Here's how the part is built. I have some questions about the finished solid (model axes, mm). A direction names the side the tool comes from. Coordinates: 2 decimals unless noted, no trailing zeros. Write each loop counter-clockwise with the first axis right and the second up, starting at its lowest first coordinate (ties: lowest second). Pieces come first, ordered by that corner, then holes.
Item 1: For faces 1 (the face through (-5, 9, 30)), 2 (the face through (-11.99, 0.53, 18.12)), 3 (the face through (0.53, 0.28, -11.99)), which set-ups out of +Z, -Z, +X, -X, +Y, -Y let a thin tool reach every point of the face, with its end or its side?
Item 2: I want a section at B-B (y = 13). Please give me the cut outline in (x, z).
Item 3: I want a section at D-D (y = 4.5). Please give me the cut outline in (x, z), and give its area (3 significant figures).
Item 4: I'm going to push flat-ended pins straight in: P1, Ø2, axis at x = 4, y = 5.5, coming from the +Z side; P2, Ø3, axis at x = -9, y = 1, coming from the -Z side; P3, Ø3, axis at x = 3.5, y = -15, coming from the -Z side; P4, Ø2, axis at x = 8.5, z = 4.5, coming from the -Y side. Where does each tip first touch, or does it pass through?
Item 5: I want a section at C-C (z = -8). Please give me the cut outline in (x, y).
Item 6: Please list where these lines run through material, in increasing order: line 1 (Y direction, x = 0, z = 13.5); line 2 (Y direction, x = 6.5, z = 25).
Item 7: I want a section at A-A (x = -4). Please give me the cut outline in (y, z).
from build123d import *

# Parameters (mm, degrees)
SKETCH_1_R          = 12
SKETCH_1_R_2        = 10
EXTRUDE_1_DEPTH     = 20
SKETCH_2_R          = 12
SKETCH_2_R_2        = 10
EXTRUDE_2_DEPTH     = 30
SKETCH_2_2_R        = 10
CUT_EXTRUDE_1_DEPTH = 30
SKETCH_1_2_R        = 10
CUT_EXTRUDE_2_DEPTH = 15


with BuildPart() as part:
    # Sketch 1 → Extrude 1 (new, symmetric)
    with BuildSketch(Plane(origin=(0, 0, 0), x_dir=(1, 0, 0), z_dir=(0, 1, 0))):
        with Locations(Location((0, 0, 0), (0, 0, 270))):
            Circle(SKETCH_1_R)
        with Locations(Location((0, 0, 0), (0, 0, 270))):
            Circle(SKETCH_1_R_2, mode=Mode.SUBTRACT)
    extrude(amount=EXTRUDE_1_DEPTH, both=True)

    # Sketch 2 → Extrude 2 (add)
    with BuildSketch(Plane.XY):
        Circle(SKETCH_2_R)
        with Locations(Location((0, 0, 0), (0, 0, 180))):
            Circle(SKETCH_2_R_2, mode=Mode.SUBTRACT)
    extrude(amount=EXTRUDE_2_DEPTH)

    # Sketch 2_2 → Cut-Extrude 1 (cut)
    with BuildSketch(Plane.XY):
        Circle(SKETCH_2_2_R)
    extrude(amount=CUT_EXTRUDE_1_DEPTH, mode=Mode.SUBTRACT)

    # Sketch 1_2 → Cut-Extrude 2 (cut, symmetric)
    with BuildSketch(Plane(origin=(0, 0, 0), x_dir=(1, 0, 0), z_dir=(0, 1, 0))):
        with Locations(Location((0, 0, 0), (0, 0, 270))):
            Circle(SKETCH_1_2_R)
    extrude(amount=CUT_EXTRUDE_2_DEPTH, both=True, mode=Mode.SUBTRACT)


solid = part.part
Answer:
1. face 1: +Z, +X, -X, +Y, -Y
1. face 2: +Z
1. face 3: none
2. outline: circle Ø24 at (0, 0); hole circle Ø20 at (0, 0)
3. outline: (-11.12, 4.5) arc R12 ccw (long way) to (11.12, 4.5) - (11.12, 30) - (8.93, 30) - (8.93, 4.5) arc R10 cw (long way) to (-8.93, 4.5) - (-8.93, 30) - (-11.12, 30) - close
3. area: 200 mm2
4. P1: stops at z = -8.66
4. P2: stops at z = -9.37
4. P3: stops at z = -11.83
4. P4: stops at y = -20
5. outline: (-8.94, -20) - (-6, -20) - (-6, 20) - (-8.94, 20) - close; (6, -20) - (8.94, -20) - (8.94, 20) - (6, 20) - close
6. line 1: y = -12 to -10, 10 to 12
6. line 2: y = -10.09 to -7.6, 7.6 to 10.09
7. outline: (-20, -11.31) - (20, -11.31) - (20, -9.17) - (-20, -9.17) - close; (-20, 9.17) - (-9.17, 9.17) - (-9.17, 30) - (-11.31, 30) - (-11.31, 11.31) - (-20, 11.31) - close; (9.17, 9.17) - (20, 9.17) - (20, 11.31) - (11.31, 11.31) - (11.31, 30) - (9.17, 30) - close
